from build123d import *

# Parameters (mm, degrees)
F0_W     = 396.858634
F0_H     = 355.6
F0_R     = 22.225
F1_DEPTH = 19.05
F2_W     = 9.525
F2_H     = 396.858634
F3_DEPTH = 9.525
F4_W     = 9.525
F4_H     = 396.858634
F5_DEPTH = 9.525


with BuildPart() as f1:
    # F0 (on Right) → F1 (new body)
    with BuildSketch(Plane.YZ):
        Rectangle(F0_W, F0_H)
        with Locations((-153.979317, -88.9)):
            Circle(F0_R, mode=Mode.SUBTRACT)
        with Locations((-51.326439, -88.9)):
            Circle(F0_R, mode=Mode.SUBTRACT)
        with Locations((51.326439, -88.9)):
            Circle(F0_R, mode=Mode.SUBTRACT)
        with Locations((153.979317, -88.9)):
            Circle(F0_R, mode=Mode.SUBTRACT)
        with Locations((-102.652878, 0)):
            Circle(F0_R, mode=Mode.SUBTRACT)
        with Locations((-153.979317, 88.9)):
            Circle(F0_R, mode=Mode.SUBTRACT)
        with Locations((-51.326439, 88.9)):
            Circle(F0_R, mode=Mode.SUBTRACT)
        Circle(F0_R, mode=Mode.SUBTRACT)
        with Locations((102.652878, 0)):
            Circle(F0_R, mode=Mode.SUBTRACT)
        with Locations((51.326439, 88.9)):
            Circle(F0_R, mode=Mode.SUBTRACT)
        with Locations((153.979317, 88.9)):
            Circle(F0_R, mode=Mode.SUBTRACT)
    extrude(amount=F1_DEPTH)

    # F2 (on face) → F3 (join)
    with BuildSketch(Plane.XY.offset(177.8)):
        with Locations((4.7625, 0)):
            Rectangle(F2_W, F2_H)
    extrude(amount=F3_DEPTH)

    # F4 (on face) → F5 (join)
    with BuildSketch(Plane(origin=(0, 0, -177.8), x_dir=(1, 0, 0), z_dir=(0, 0, -1))):
        with Locations((4.7625, 0)):
            Rectangle(F4_W, F4_H)
    extrude(amount=F5_DEPTH)


solid = f1.part
Verification items for the finished model (mm, model axes). A direction names the side the tool comes from. Give positions to 0.01 mm unless a question says otherwise; leave off trailing zeros. Write each loop counter-clockwise with the first axis right and the second up, starting at its lowest first coordinate (ties: lowest second). Pieces come first, ordered by that corner, then holes. Notation, with made-up numbers: M 20,38.25 L 65,38.25 A21 cw 65,44.25 Z; hole C 25.25,-31.5 d9. An arc over 180 degrees is marked long. Use CSV: the item, a comma, the result in double quotes.
1) Go/stop test with flat-tipped pins: pin 1 Ø5 at (x, y) = (16.5, -84) entering from +Z; pin 2 Ø8 at (y, z) = (73, 87) entering from +X; pin 3 Ø5 at (x, y) = (13.5, 6) entering from -Z; pin 4 Ø3 at (y, z) = (-86, 181) entering from +X (3 decimals). Record where each tip stops, or that it passes through.
Final values:
pin 1,"z = 177.8"
pin 2,"x = 19.05"
pin 3,"z = -177.8"
pin 4,"x = 9.525"
2) Access from +Z, -Z, +X, -X, +Y, -Y to the whole of each face (thin tool, end or side, straight path). Record for faces 1 (the face through (9.525, 3, -182)), 2 (the face through (14, -3, 177.8)), 3 (the face through (9.392, -81.454, 6.676)).
Final values:
face 1,"-Z, +X, +Y, -Y"
face 2,"+Z, +X, +Y, -Y"
face 3,"+X, -X"
3) Cross-section at C-C (y = 104.5). Enter the section's corners in (x, z) (3 decimals), plus the area to 3 significant figures.
Final values:
outline,"M 0,-187.325 L 9.525,-187.325 L 9.525,-177.8 L 19.05,-177.8 L 19.05,-22.148 L 0,-22.148 Z; M 0,22.148 L 19.05,22.148 L 19.05,177.8 L 9.525,177.8 L 9.525,187.325 L 0,187.325 Z"
area,"6,110 mm²"
4) Cross-section at D-D (z = 0). Enter the section's corners in (x, y) (3 decimals).
Final values:
outline,"M 0,-198.429 L 19.05,-198.429 L 19.05,-124.878 L 0,-124.878 Z; M 0,-80.428 L 19.05,-80.428 L 19.05,-22.225 L 0,-22.225 Z; M 0,22.225 L 19.05,22.225 L 19.05,80.428 L 0,80.428 Z; M 0,124.878 L 19.05,124.878 L 19.05,198.429 L 0,198.429 Z"
5) Cross-section at A-A (z = 88.9). Enter the section's corners in (x, y), plus the area to 3 significant figures.
Final values:
outline,"M 0,-198.43 L 19.05,-198.43 L 19.05,-176.2 L 0,-176.2 Z; M 0,-131.75 L 19.05,-131.75 L 19.05,-73.55 L 0,-73.55 Z; M 0,-29.1 L 19.05,-29.1 L 19.05,29.1 L 0,29.1 Z; M 0,73.55 L 19.05,73.55 L 19.05,131.75 L 0,131.75 Z; M 0,176.2 L 19.05,176.2 L 19.05,198.43 L 0,198.43 Z"
area,"4,170 mm²"
6) Material ranges on line 1 along Y through (x, z) = (7, -89.5); line 2 along Z through (x, y) = (1, -48) (3 decimals); line 3 along Z through (x, y) = (1.5, 70) (3 decimals), recorded low to high.
Final values:
line 1,"-198.43 to -176.2, -131.76 to -73.54, -29.11 to 29.11, 73.54 to 131.76, 176.2 to 198.43"
line 2,"-187.325 to -110.875, -66.925 to 66.925, 110.875 to 187.325"
line 3,"-187.325 to -100.952, -76.848 to 76.848, 100.952 to 187.325"
7) Cross-section at B-B (x = 6). State how many separate pieces and enclosed holes the cut face has, plus the area to 3 significant figures.
Final values:
separate pieces,"1"
enclosed holes,"11"
area,"132,000 mm²"
8) Release check for a two-part mould opening along Z. For faces 4 (the face through (9, 198.429, 3)), 5 (the face through (5, -3, -187.325)), 6 (the face through (9.39, 137.6, -73.88)) record: released by +Z, released by -Z, zero draft, split by the parting line, or undercut.
Final values:
face 4,"zero draft"
face 5,"released by -Z"
face 6,"undercut"
